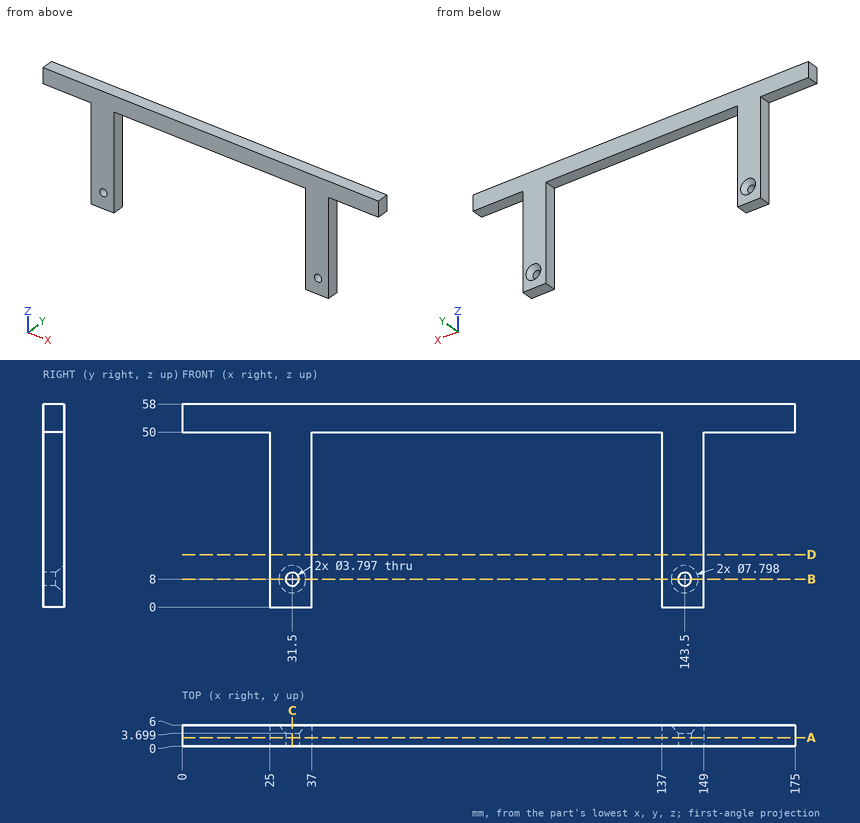
The figure shows three views and two pictorial views of one solid part (mm, origin at its lowest corner). Answer the questions. Give positions to 0.01 mm unless a question says otherwise; leave off trailing zeros. Order: outer loops, then holes, each group sorted by start corner. A loop starts at its lowest first (then second) coordinate and runs counter-clockwise, first axis right, second up. Notation, with made-up numbers: (-11.5, -22.75) -> (33.5, -22.75) arc R26 ccw to (33.5, 9.25) -> close; hole circle Ø3 at (7.5, -31.5). An arc over 180 degrees is marked (long way). Answer as a JSON object with one key per item and string values. Group by question number.
Item 1: The part is cut by section A-A on y = 2.45. Write down the section's boundary in (x, z), and give its area (3 significant figures).
Item 2: The part is cut by section B-B on z = 8. Write down the section's boundary in (x, y).
Item 3: Consider L1, parallel to X at y = 1.85, z = 8; L2, parallel to X at y = 1.5, z = 44; L3, parallel to Z at x = 31.5, y = 1.65. Determine where each line is inside the solid, lowest interval first. Write a range as from..to.
Item 4: The part is cut by section D-D on z = 15. Write down the section's boundary in (x, y).
Item 5: The part is cut by section C-C on x = 31.5. Write down the section's boundary in (y, z), and give its area (3 significant figures).
Item 6: Flat-ended cylindrical pins translate along their axes: pin 1 (1.8 mm diameter, centred on y = 2.5, z = 34.5, fed in from -X); pin 2 (3 mm diameter, centred on x = 95, y = 3, fed in from -Z); pin 3 (1.8 mm diameter, centred on y = 4.5, z = 25.5, fed in from +X). Find the tip coordinate at first contact, or state that the pin passes through.
Result set:
{
 "1": {"outline": "(0, 50) -> (25, 50) -> (25, 0) -> (37, 0) -> (37, 50) -> (137, 50) -> (137, 0) -> (149, 0) -> (149, 50) -> (175, 50) -> (175, 58) -> (0, 58) -> close; hole circle Ø3.8 at (31.5, 8); hole circle Ø3.8 at (143.5, 8)", "area": "2,580 mm²"},
 "2": {"outline": "(25, 0) -> (29.6, 0) -> (29.6, 3.7) -> (27.6, 6) -> (25, 6) -> close; (33.4, 0) -> (37, 0) -> (37, 6) -> (35.4, 6) -> (33.4, 3.7) -> close; (137, 0) -> (141.6, 0) -> (141.6, 3.7) -> (139.6, 6) -> (137, 6) -> close; (145.4, 0) -> (149, 0) -> (149, 6) -> (147.4, 6) -> (145.4, 3.7) -> close"},
 "3": {"L1": "25..29.6, 33.4..37, 137..141.6, 145.4..149", "L2": "25..37, 137..149", "L3": "0..6.1, 9.9..58"},
 "4": {"outline": "(25, 0) -> (37, 0) -> (37, 6) -> (25, 6) -> close; (137, 0) -> (149, 0) -> (149, 6) -> (137, 6) -> close"},
 "5": {"outline": "(0, 0) -> (6, 0) -> (6, 4.1) -> (3.7, 6.1) -> (0, 6.1) -> close; (0, 9.9) -> (3.7, 9.9) -> (6, 11.9) -> (6, 58) -> (0, 58) -> close", "area": "321 mm²"},
 "6": {"pin 1": "x = 25", "pin 2": "z = 50", "pin 3": "x = 149"}
}
